```python
from build123d import *
from build123d.topology import SkipClean

# Parameters (mm, degrees)
BOSS_EXTRU_1_DEPTH      = 5.8
ESQUISSE2_R             = 1.5
ESQUISSE2_R_2           = 6.4
ENL_V_MAT_EXTRU_1_DEPTH = 5.8
ESQUISSE3_W             = 42
ESQUISSE3_H             = 20.5
ENL_V_MAT_EXTRU_2_DEPTH = 5.8


with BuildPart() as part:
    # Esquisse1 → Boss.-Extru.1 (new body)
    with BuildSketch(Plane(origin=(0, 0, 0), x_dir=(1, 0, 0), z_dir=(0, 1, 0))):
        Polygon((0, 0), (-18.5, 0), (-18.5, -33), (-73.3, -73.793956851), (-59.8, -85.241227268), (-40.8, -119.3), (-36.8, -119.3), (-36.8, -68.3), (0, -68.3), align=None)
    boss_extru_1 = extrude(amount=BOSS_EXTRU_1_DEPTH)

    # Esquisse2 → Enlèv. mat.-Extru.1 (cut)
    with BuildSketch(Plane(origin=(0, 5.8, 0), x_dir=(1, 0, 0), z_dir=(0, 1, 0))):
        with Locations(Location((-13.5, -5, 0), (0, 0, 270))):
            Circle(ESQUISSE2_R)
        with Locations((0, -19)):
            Circle(ESQUISSE2_R_2)
        with Locations(Location((-13.5, -32, 0), (0, 0, 270))):
            Circle(ESQUISSE2_R)
    enl_v_mat_extru_1 = extrude(amount=-ENL_V_MAT_EXTRU_1_DEPTH, mode=Mode.SUBTRACT)

    # Symétrie2: Boss.-Extru.1, Enlèv. mat.-Extru.1 across plane
    with SkipClean():  # the faces are left unmerged after this step: merging them gives an invalid solid
        add(boss_extru_1.mirror(Plane(origin=(0, 5.8, 68.3), x_dir=(0, 0, 1), z_dir=(-1, 0, 0))))
        add(enl_v_mat_extru_1.mirror(Plane(origin=(0, 5.8, 68.3), x_dir=(0, 0, 1), z_dir=(-1, 0, 0))), mode=Mode.SUBTRACT)

    # Esquisse3 → Enlèv. mat.-Extru.2 (cut)
    with SkipClean():  # the faces are left unmerged after this step: merging them gives an invalid solid
        with BuildSketch(Plane(origin=(0, 5.8, 0), x_dir=(1, 0, 0), z_dir=(0, 1, 0))):
            with Locations((-10.1, -55.25)):
                Rectangle(ESQUISSE3_W, ESQUISSE3_H)
        extrude(amount=-ENL_V_MAT_EXTRU_2_DEPTH, mode=Mode.SUBTRACT)


solid = part.part
```
Input: part model. Units: mm. Frame: model coordinates. A direction names the side the tool comes from. Coordinates: 2 decimals unless noted, no trailing zeros. Write each loop counter-clockwise with the first axis right and the second up, starting at its lowest first coordinate (ties: lowest second). Pieces come first, ordered by that corner, then holes.
1) Section D-D on z = 78. Output: boundary loops of the cut face in (x, y), and give its area (3 significant figures).
2) Material intervals for line 1 along X through (y, z) = (4.6, 32); line 2 along Z through (x, y) = (-9, 2.95); line 3 along Z through (x, y) = (-2.5, 3.65), sorted ascending.
3) Pin query (flat end, axial travel): pin 1 Ø3 at (y, z) = (3, 24) entering from -X; pin 2 Ø1.7 at (x, y) = (-8, 3.5) entering from +Z; pin 3 Ø2 at (x, y) = (42.5, 3) entering from -Z; pin 4 Ø2.5 at (x, z) = (13.5, 32) entering from -Y. Return the tip coordinate at first contact, or that it passes through.
4) Set-up query: faces 1 (the flat face through (-31.1, 3, 55)), 2 (the flat face through (-39, 3, 119.3)), 3 (the flat face through (1, 3, 68.3)). Return all of +Z, -Z, +X, -X, +Y, -Y with unobstructed straight access to the full face (end or side cutting, diameter ignored); none if empty.
5) Mould query, pull axis X, two halves, no side actions, for faces 4 (the flat face through (-10, 3, 45)), 5 (the flat face through (0, 5.8, 68)), 6 (the flat face through (18.5, 3, 16)). Classes: pulls with the +X half, pulls with the -X half, needs draft (parallel to the pull), parting line crosses it, or undercut.
6) Section B-B on z = 19. Output: boundary loops of the cut face in (x, y), and give its area (3 significant figures).
7) Section A-A on x = 0. Output: boundary loops of the cut face in (y, z), and give its area (3 significant figures).
8) Section C-C on y = 4.8. Output: boundary loops of the cut face in (x, z).
Check result:
1. outline: (-68.34, 0) - (-36.8, 0) - (-36.8, 5.8) - (-68.34, 5.8) - close; (36.8, 0) - (68.34, 0) - (68.34, 5.8) - (36.8, 5.8) - close
1. area: 366 mm2
2. line 1: x = -18.5 to -15, -12 to 12, 15 to 18.5
2. line 2: z = 0 to 45, 65.5 to 68.3
2. line 3: z = 0 to 13.11, 24.89 to 45, 65.5 to 68.3
3. pin 1: stops at x = -18.5
3. pin 2: stops at z = 68.3
3. pin 3: stops at z = 50.12
3. pin 4: passes through
4. face 1: +Y, -Y
4. face 2: +Z, +X, -X, +Y, -Y
4. face 3: +Z, +Y, -Y
5. face 4: undercut
5. face 5: needs draft
5. face 6: pulls with the +X half
6. outline: (-18.5, 0) - (-6.4, 0) - (-6.4, 5.8) - (-18.5, 5.8) - close; (6.4, 0) - (18.5, 0) - (18.5, 5.8) - (6.4, 5.8) - close
6. area: 140 mm2
7. outline: (0, 0) - (5.8, 0) - (5.8, 12.6) - (0, 12.6) - close; (0, 25.4) - (5.8, 25.4) - (5.8, 45) - (0, 45) - close; (0, 65.5) - (5.8, 65.5) - (5.8, 68.3) - (0, 68.3) - close
7. area: 203 mm2
8. outline: (-73.3, 73.79) - (-18.5, 33) - (-18.5, 0) - (18.5, 0) - (18.5, 33) - (73.3, 73.79) - (59.8, 85.24) - (40.8, 119.3) - (36.8, 119.3) - (36.8, 68.3) - (-36.8, 68.3) - (-36.8, 119.3) - (-40.8, 119.3) - (-59.8, 85.24) - close; hole (-31.1, 45) - (10.9, 45) - (10.9, 65.5) - (-31.1, 65.5) - close; hole circle Ø3 at (-13.5, 5); hole circle Ø3 at (-13.5, 32); hole circle Ø12.8 at (0, 19); hole circle Ø3 at (13.5, 5); hole circle Ø3 at (13.5, 32)
